Source: CAD feature listing. Evaluate the final solid. Frame: model axes, mm. A direction names the side the tool comes from. Give positions to 0.01 mm unless a question says otherwise; leave off trailing zeros. Write each loop counter-clockwise with the first axis right and the second up, starting at its lowest first coordinate (ties: lowest second). Pieces come first, ordered by that corner, then holes. Notation, with made-up numbers: M -12,-2.5 L 25,-2.5 A22 ccw 25,31.5 Z; hole C 76,41 d7. An arc over 180 degrees is marked long. Return JSON: item names as keys, results as strings.
```python
from build123d import *

# Parameters (mm, degrees)
SKETCH1_W           = 227.6
SKETCH1_H           = 30
SKETCH1_R           = 0.5
SKETCH1_R_2         = 5
SKETCH1_R_3         = 1.1
SKETCH1_W_2         = 24
SKETCH1_H_2         = 14
BOSS_EXTRUDE1_DEPTH = 10


with BuildPart() as part:
    # Sketch1 → Boss-Extrude1 (new body)
    with BuildSketch(Plane.XY):
        with Locations((113.8, 15)):
            Rectangle(SKETCH1_W, SKETCH1_H)
        with Locations((35, 7.47)):
            Circle(SKETCH1_R, mode=Mode.SUBTRACT)
        with Locations((21.47, 15)):
            Circle(SKETCH1_R, mode=Mode.SUBTRACT)
        with Locations((35, 15)):
            Circle(SKETCH1_R_2, mode=Mode.SUBTRACT)
        with Locations((48.53, 15)):
            Circle(SKETCH1_R, mode=Mode.SUBTRACT)
        with Locations((35, 22.53)):
            Circle(SKETCH1_R, mode=Mode.SUBTRACT)
        with Locations((219.5, 15)):
            Circle(SKETCH1_R_3, mode=Mode.SUBTRACT)
        with Locations((191.7, 15)):
            Circle(SKETCH1_R_3, mode=Mode.SUBTRACT)
        with Locations((205.6, 15)):
            Rectangle(SKETCH1_W_2, SKETCH1_H_2, mode=Mode.SUBTRACT)
    extrude(amount=BOSS_EXTRUDE1_DEPTH)


solid = part.part
```
1) Draft query along X for faces 1 (the face through (112, 0, 5)), 2 (the face through (205, 22, 5)), 3 (the face through (0, 15, 5)). Return one class per face: released by +X, released by -X, zero draft, split by the parting line, or undercut.
Numbers:
{"face 1": "zero draft", "face 2": "undercut", "face 3": "released by -X"}
2) Set-up query: faces 4 (the face through (227.6, 15, 5)), 5 (the face through (193.6, 15, 5)). Return all of +Z, -Z, +X, -X, +Y, -Y with unobstructed straight access to the full face (end or side cutting, diameter ignored); none if empty.
Numbers:
{"face 4": "+Z, -Z, +X, +Y, -Y", "face 5": "+Z, -Z"}
3) Cut plane A-A, the plane x = 197. Return the cut outline in (y, z).
Numbers:
{"outline": "M 0,0 L 8,0 L 8,10 L 0,10 Z; M 22,0 L 30,0 L 30,10 L 22,10 Z"}
4) Cut plane B-B, the plane z = 8. Give the number of separate pieces and of enclosed holes in the cut face, then the cut area to 3 significant figures.
Numbers:
{"separate pieces": "1", "enclosed holes": "8", "area": "6,400 mm²"}
5) Line query: line 1 (Y direction, x = 35, z = 4.25); line 2 (Y direction, x = 219.5, z = 3.5); line 3 (X direction, y = 12.75, z = 2.5). Output: solid intervals per line, ascending. Write a range as [from, to].
Numbers:
{"line 1": "y = [0, 6.97], [7.97, 10], [20, 22.03], [23.03, 30]", "line 2": "y = [0, 13.9], [16.1, 30]", "line 3": "x = [0, 30.53], [39.47, 193.6], [217.6, 227.6]"}
